For this review, take the finished solid that the model builds, in its own axes (mm). A direction names the side the tool comes from. Round coordinates to 2 decimals unless told otherwise and drop trailing zeros. Loops run counter-clockwise (first coordinate to the right, second up) from the corner with the lowest first, then second, coordinate; pieces in that order, holes last. Notation, with made-up numbers: (-36, -23.75) -> (-3, -23.75) arc R21 cw to (-3, -7.75) -> close; hole circle Ø4 at (64.5, -33). An arc over 180 degrees is marked (long way). Write each question's results on one line, items separated by ' | '.
```python
from build123d import *

# Parameters (mm, degrees)
SKETCH2_R               = 9.61
SKETCH2_R_2             = 3.985714286
SKETCH2_R_3             = 1.55
BOSS_EXTRUDE2_DEPTH     = 7
SKETCH3_R               = 4.5
BOSS_EXTRUDE3_DEPTH     = 3
SKETCH4_R               = 4.5
CUT_EXTRUDE1_DEPTH      = 6
CHAMFER3_SIZE           = 1
BOSS_EXTRUDE4_START     = -3
BOSS_EXTRUDE4_OUTLINE_R = 1.55
BOSS_EXTRUDE4_DEPTH     = 3


# Read off the part's stored shape, not the designer's step: Boss-Extrude4
with BuildPart() as part:
    # Sketch2 → Boss-Extrude2 (new body)
    with BuildSketch(Plane.XY.offset(-179.459781676)):
        Circle(SKETCH2_R)
        Circle(SKETCH2_R_2, mode=Mode.SUBTRACT)
        with Locations((6.731428571, 0)):
            Circle(SKETCH2_R_3, mode=Mode.SUBTRACT)
        with Locations((-6.731428571, 0)):
            Circle(SKETCH2_R_3, mode=Mode.SUBTRACT)
    extrude(amount=BOSS_EXTRUDE2_DEPTH)

    # Sketch3 → Boss-Extrude3 (add)
    with BuildSketch(Plane(origin=(0, 0, -179.459781676), x_dir=(-1, 0, 0), z_dir=(0, 0, -1))):
        Circle(SKETCH3_R)
    extrude(amount=-BOSS_EXTRUDE3_DEPTH)

    # Sketch4 → Cut-Extrude1 (cut)
    with BuildSketch(Plane.XY.offset(-176.459781676)):
        Circle(SKETCH4_R)
    extrude(amount=-CUT_EXTRUDE1_DEPTH, mode=Mode.SUBTRACT)

    # Chamfer3
    chamfer3_edges = [part.edges().sort_by_distance(p)[0] for p in [
        (-3.985714286, 0, -172.459781676),
    ]]
    chamfer(chamfer3_edges, length=CHAMFER3_SIZE)

    # Boss-Extrude4 outline → Boss-Extrude4 (add)
    with BuildSketch(Plane.XY.offset(-172.459781676).offset(BOSS_EXTRUDE4_START)):
        with Locations((6.731428571, 0)):
            Circle(BOSS_EXTRUDE4_OUTLINE_R)
        with Locations((-6.731428571, 0)):
            Circle(BOSS_EXTRUDE4_OUTLINE_R)
    extrude(amount=BOSS_EXTRUDE4_DEPTH)


solid = part.part
```
1. Consider section C-C (z = -177.5). State the section outline as (x, y) points, plus the area to 3 significant figures.
Values found:
outline: circle Ø19.22 at (0, 0); hole circle Ø3.1 at (-6.73, 0); hole circle Ø9 at (0, 0); hole circle Ø3.1 at (6.73, 0) | area: 211 mm2
2. Consider section A-A (x = 0). State the section outline as (y, z) points.
Values found:
outline: (-9.61, -179.46) -> (-4.5, -179.46) -> (-4.5, -176.46) -> (-3.99, -176.46) -> (-3.99, -173.46) -> (-4.99, -172.46) -> (-9.61, -172.46) -> close; (3.99, -176.46) -> (4.5, -176.46) -> (4.5, -179.46) -> (9.61, -179.46) -> (9.61, -172.46) -> (4.99, -172.46) -> (3.99, -173.46) -> close
3. To check wall thickness, follow probe 1 along Y at (x, z) = (0, -178.6); probe 2 along X at (y, z) = (-0.5, -177); probe 3 along Y at (x, z) = (0, -174.35). State the ranges of each line that lie inside material, in increasing order.
Values found:
probe 1: y = -9.61 to -4.5, 4.5 to 9.61 | probe 2: x = -9.6 to -8.2, -5.26 to -4.47, 4.47 to 5.26, 8.2 to 9.6 | probe 3: y = -9.61 to -3.99, 3.99 to 9.61
4. Draft analysis for pull direction X (two halves, no side actions). For faces 1 (the face through (7, 0, -175.46)), 2 (the face through (-2.083, -9.381, -176.009)), 3 (the face through (4.1, 2.3, -179.46)), 4 (the face through (5.5, -0.94, -177.49)), state which applies: released by +X, released by -X, zero draft, split by the parting line, or undercut.
Values found:
face 1: undercut | face 2: split by the parting line | face 3: zero draft | face 4: undercut
5. Tool access review of faces 5 (the face through (-0.59, 4.46, -177.94)), 6 (the face through (-0.86, -3.89, -174.98)): name each direction out of +Z, -Z, +X, -X, +Y, -Y from which nothing blocks a thin tool from reaching the whole face with its end or side.
Values found:
face 5: -Z | face 6: +Z, -Z
6. For pin 1 (1 mm diameter, centred on y = -5, z = -176, fed in from -X); pin 2 (1.5 mm diameter, centred on x = -3.5, z = -176, fed in from +Y); pin 3 (1.6 mm diameter, centred on x = -7, y = 0.5, fed in from -Z); pin 4 (5 mm diameter, centred on x = 0, y = 0, fed in from -Z), all flat-tipped, find the tip position at first contact; note any pin that passes through.
Values found:
pin 1: stops at x = -8.49 | pin 2: stops at y = 9.21 | pin 3: stops at z = -175.46 | pin 4: passes through
7. Consider section B-B (y = 0). State the section outline as (x, z) points, plus the area to 3 significant figures.
Values found:
outline: (-9.61, -179.46) -> (-8.28, -179.46) -> (-8.28, -175.46) -> (-5.18, -175.46) -> (-5.18, -179.46) -> (-4.5, -179.46) -> (-4.5, -176.46) -> (-3.99, -176.46) -> (-3.99, -173.46) -> (-4.99, -172.46) -> (-9.61, -172.46) -> close; (3.99, -176.46) -> (4.5, -176.46) -> (4.5, -179.46) -> (5.18, -179.46) -> (5.18, -175.46) -> (8.28, -175.46) -> (8.28, -179.46) -> (9.61, -179.46) -> (9.61, -172.46) -> (4.99, -172.46) -> (3.99, -173.46) -> close | area: 49.9 mm2
8. Consider section D-D (x = -7.5). State the section outline as (y, z) points.
Values found:
outline: (-6.01, -179.46) -> (-1.35, -179.46) -> (-1.35, -175.46) -> (1.35, -175.46) -> (1.35, -179.46) -> (6.01, -179.46) -> (6.01, -172.46) -> (-6.01, -172.46) -> close
